from build123d import *

# Parameters (mm, degrees)
SKETCH1_R           = 3.75
SKETCH1_R_2         = 3
BOSS_EXTRUDE1_DEPTH = 4
BOSS_EXTRUDE2_START = 6
SKETCH2_R           = 3.75
SKETCH2_R_2         = 1
BOSS_EXTRUDE2_DEPTH = 6
BOSS_EXTRUDE3_START = 1
SKETCH3_R           = 2
SKETCH3_R_2         = 1
BOSS_EXTRUDE3_DEPTH = 1


with BuildPart() as part:
    # Sketch1 → Boss-Extrude1 (new body)
    with BuildSketch(Plane.XY):
        Circle(SKETCH1_R)
        Circle(SKETCH1_R_2, mode=Mode.SUBTRACT)
    extrude(amount=BOSS_EXTRUDE1_DEPTH)

    # Sketch2 → Boss-Extrude2 (add)
    with BuildSketch(Plane(origin=(0, 0, 0), x_dir=(-1, 0, 0), z_dir=(0, 0, -1)).offset(BOSS_EXTRUDE2_START)):
        Circle(SKETCH2_R)
        Circle(SKETCH2_R_2, mode=Mode.SUBTRACT)
    extrude(amount=-BOSS_EXTRUDE2_DEPTH)

    # Sketch3 → Boss-Extrude3 (add)
    with BuildSketch(Plane(origin=(0, 0, -6), x_dir=(-1, 0, 0), z_dir=(0, 0, -1)).offset(BOSS_EXTRUDE3_START)):
        Circle(SKETCH3_R)
        Circle(SKETCH3_R_2, mode=Mode.SUBTRACT)
    extrude(amount=-BOSS_EXTRUDE3_DEPTH)


solid = part.part
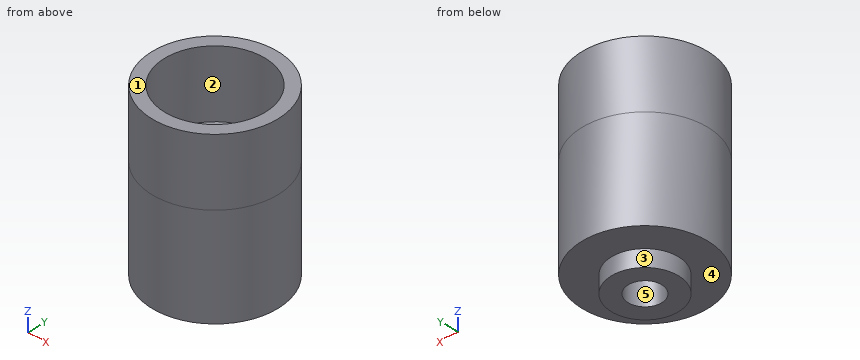
Verification items for the finished model (mm, model axes). Face numbers are marked on the shaded views. A direction names the side the tool comes from. Coordinates: 2 decimals unless noted, no trailing zeros. Order: outer loops, then holes, each group sorted by start corner. A loop starts at its lowest first (then second) coordinate and runs counter-clockwise, first axis right, second up.
1. Go/stop test with flat-tipped pins: pin 1 Ø2 at (y, z) = (2, 2) entering from -X; pin 2 Ø3 at (y, z) = (-2, 0.5) entering from -X; pin 3 Ø1.6 at (x, y) = (0, 0) entering from +Z; pin 4 Ø1.5 at (x, z) = (1, -3) entering from -Y. Record where each tip stops, or that it passes through.
Results found:
pin 1: stops at x = -3.61
pin 2: stops at x = -3.72
pin 3: passes through
pin 4: stops at y = -3.74
2. Sectioned sample at C-C, the plane z = 1.25. Record the cut outline in (x, y), and give its area (3 significant figures).
Results found:
outline: circle Ø7.5 at (0, 0); hole circle Ø6 at (0, 0)
area: 15.9 mm2
3. Scan lines: line 1 (Y direction, x = 0, z = -1.75); line 2 (Y direction, x = 0, z = 2.6); line 3 (Z direction, x = 0.5, y = 1). Record each from-to range of solid material in increasing order.
Results found:
line 1: y = -3.75 to -1, 1 to 3.75
line 2: y = -3.75 to -3, 3 to 3.75
line 3: z = -7 to 0
4. Sectioned sample at A-A, the plane y = 0. Record the cut outline in (x, z), and give its area (3 significant figures).
Results found:
outline: (-3.75, -6) - (-2, -6) - (-2, -7) - (-1, -7) - (-1, 0) - (-3, 0) - (-3, 4) - (-3.75, 4) - close; (1, -7) - (2, -7) - (2, -6) - (3.75, -6) - (3.75, 4) - (3, 4) - (3, 0) - (1, 0) - close
area: 41.0 mm2
5. Set-up check for the marked faces 4 and 5: record each of +Z, -Z, +X, -X, +Y, -Y from which the full face is reachable in a straight line by a thin tool's end or side.
Results found:
face 4: -Z
face 5: +Z, -Z
6. Release check for a two-part mould opening along Y. For the marked faces 1, 2 and 3 record: +Y half, -Y half, draft (parallel to the pull), parting line (faces both ways), or undercut.
Results found:
face 1: draft
face 2: undercut
face 3: parting line
7. Sectioned sample at D-D, the plane y = 1.25. Record the cut outline in (x, z), and give its area (3 significant figures).
Results found:
outline: (-3.54, -6) - (-1.56, -6) - (-1.56, -7) - (1.56, -7) - (1.56, -6) - (3.54, -6) - (3.54, 4) - (2.73, 4) - (2.73, 0) - (-2.73, 0) - (-2.73, 4) - (-3.54, 4) - close
area: 52.0 mm2
